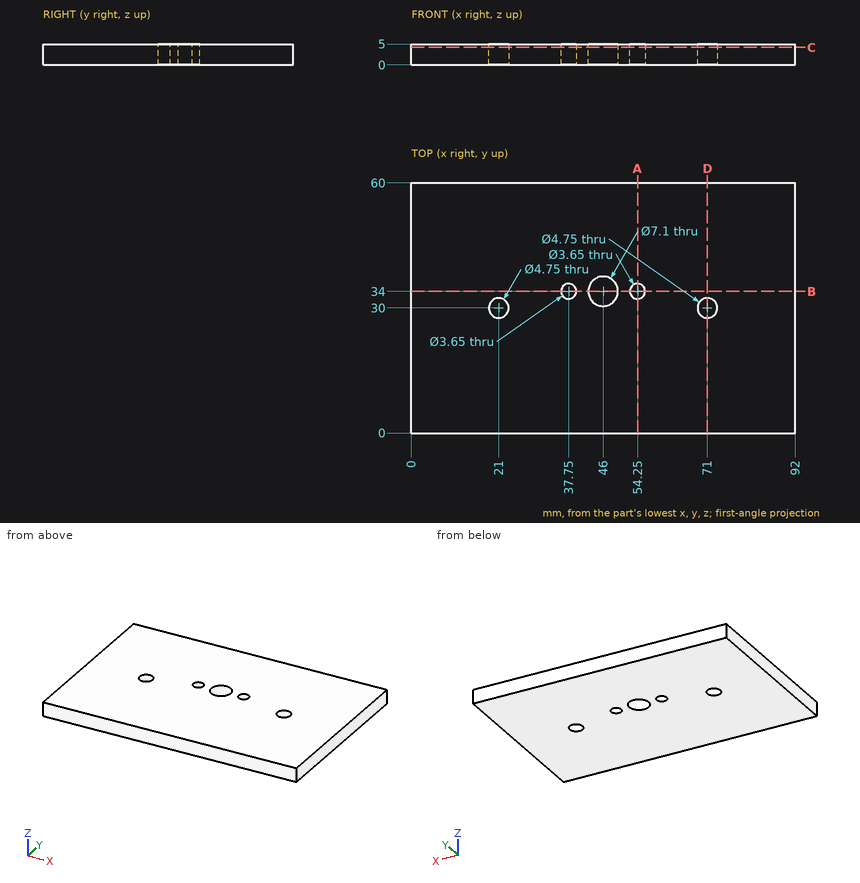
Design review of the part shown in the three views and the two pictorial views. Dimensions are in mm from the part's minimum x, y and z. Round coordinates to 2 decimals unless told otherwise and drop trailing zeros. Loops run counter-clockwise (first coordinate to the right, second up) from the corner with the lowest first, then second, coordinate; pieces in that order, holes last. Notation, with made-up numbers: M 41,-16.5 L 68,-16.5 A20 cw 68,12.5 Z; hole C 50,-35.75 d3. An arc over 180 degrees is marked long. Put each result on its own line as item: value.
Q1. To check wall thickness, follow L1, parallel to Y at x = 21, z = 2.05 (3 decimals); L2, parallel to Y at x = 46, z = 3.15. State the ranges of each line that lie inside material, in increasing order.
Result set:
L1: y = 0 to 27.625, 32.375 to 60
L2: y = 0 to 30.45, 37.55 to 60
Q2. Consider section A-A, the plane x = 54.25. Give the boundary of the cut face in (y, z) (3 decimals), then the cut area to 3 significant figures.
Result set:
outline: M 0,0 L 32.175,0 L 32.175,5 L 0,5 Z; M 35.825,0 L 60,0 L 60,5 L 35.825,5 Z
area: 282 mm²
Q3. Consider section D-D, the plane x = 71. Give the boundary of the cut face in (y, z) (3 decimals), then the cut area to 3 significant figures.
Result set:
outline: M 0,0 L 27.625,0 L 27.625,5 L 0,5 Z; M 32.375,0 L 60,0 L 60,5 L 32.375,5 Z
area: 276 mm²
Q4. Consider section C-C, the plane z = 4.2. Give the boundary of the cut face in (x, y) (3 decimals).
Result set:
outline: M 0,0 L 92,0 L 92,60 L 0,60 Z; hole C 21,30 d4.75; hole C 37.75,34 d3.65; hole C 46,34 d7.1; hole C 54.25,34 d3.65; hole C 71,30 d4.75
Q5. Consider section B-B, the plane y = 34. Give the boundary of the cut face in (x, z) (3 decimals), then the cut area to 3 significant figures.
Result set:
outline: M 0,0 L 35.925,0 L 35.925,5 L 0,5 Z; M 39.575,0 L 42.45,0 L 42.45,5 L 39.575,5 Z; M 49.55,0 L 52.425,0 L 52.425,5 L 49.55,5 Z; M 56.075,0 L 92,0 L 92,5 L 56.075,5 Z
area: 388 mm²
Q6. For pin 1 (3 mm diameter, centred on x = 21, y = 30, fed in from -Z), flat-tipped, find the tip position at first contact; note if it passes through.
Result set:
pin 1: passes through
